Can you work these out from the model? Positions are in its coordinate system, mm. A direction names the side the tool comes from. Round coordinates to 2 decimals unless told otherwise and drop trailing zeros. Write each loop counter-clockwise with the first axis right and the second up, starting at its lowest first coordinate (ties: lowest second). Pieces come first, ordered by that corner, then holes.
Q1. Please list where these lines run through material, in increasing order: line 1 along Y through (x, z) = (-4.25, -0.75); line 2 along Y through (x, z) = (-9, -0.45); line 3 along Z through (x, y) = (4, -7.5).
Q2. For faces 1 (the conical face through (12.996, -13.063, -0.285)), 2 (the flat face through (-0.508, 2.215, -0.493)), which set-ups out of +Z, -Z, +X, -X, +Y, -Y let a thin tool reach every point of the face, with its end or its side?
Q3. If we section it at B-B (x = 5): Please give me the cut outline in (y, z), plus the area to 3 significant figures.
Q4. I'm going to push flat-ended pins straight in: pin 1 Ø8 at (x, y) = (2.5, 6) entering from +Z; pin 2 Ø0.5 at (y, z) = (7, -0.5) entering from -X; pin 3 Ø0.5 at (y, z) = (-5, -0.5) entering from +X; pin 4 Ø0.8 at (y, z) = (5, -0.5) entering from +X. Where does each tip first touch, or does it pass through?
Q5. If we section it at C-C (z = -1.5): Please give me the cut outline in (x, y).
Q6. If we section it at D-D (x = -8.25): Please give me the cut outline in (y, z).
Q7. If we section it at A-A (y = 2.25): Please give me the cut outline in (x, z), plus the area to 3 significant figures.
Q8. We'd pull the mould along X, two halves only. Please class faces 3 (the flat face through (-0.24, -2.57, -0.49)), 4 (the cylindrical face through (13, 14, -3)), 5 (the cylindrical face through (-13, -14, -3)), 6 (the flat face through (0, 3, 0)): +X half, -X half, draft (parallel to the pull), parting line (faces both ways), or undercut.
from build123d import *

# Parameters (mm, degrees)
SKETCH1_W             = 30
SKETCH1_H             = 30
BOSS_EXTRUDE1_DEPTH   = 5
SKETCH1_3_OUTSIDE_W   = 40.544
SKETCH1_3_OUTSIDE_H   = 40.544
SKETCH1_3_OUTSIDE_W_2 = 30
SKETCH1_3_OUTSIDE_H_2 = 30
CUT_EXTRUDE1_DEPTH    = 1
FILLET1_R             = 5
CHAMFER1_SIZE         = 1


with BuildPart() as part:
    # Sketch1 → Boss-Extrude1 (new body)
    with BuildSketch(Plane(origin=(0, 0, 0), x_dir=(0, 1, 0), z_dir=(0, 0, 1))):
        Rectangle(SKETCH1_W, SKETCH1_H)
    extrude(amount=-BOSS_EXTRUDE1_DEPTH)

    # Sketch1<3> outside → Cut-Extrude1 (cut)
    # profile 1 of 2: a face of its own
    with BuildSketch(Plane(origin=(0, 0, 0), x_dir=(0, 1, 0), z_dir=(0, 0, 1))):
        Rectangle(SKETCH1_3_OUTSIDE_W, SKETCH1_3_OUTSIDE_H)
        Rectangle(SKETCH1_3_OUTSIDE_W_2, SKETCH1_3_OUTSIDE_H_2, mode=Mode.SUBTRACT)
    # profile 2 of 2: a face of its own
    with BuildSketch(Plane(origin=(0, 0, 0), x_dir=(0, 1, 0), z_dir=(0, 0, 1))):
        Polygon((7.730978261, -10), (5.072463768, -10), (4.769021739, 2.68115942), (4.637681159, 7.232789855), (3.691123188, 4.524456522), (0.697463768, -3.623188406), (-1.186594203, -3.623188406), (-3.994565217, 4.216485507), (-4.927536232, 7.232789855), (-4.990942029, 2.463768116), (-5.362318841, -10), (-7.930253623, -10), (-6.933876812, 10), (-3.704710145, 10), (-1.014492754, 2.255434783), (-0.144927536, -0.357789855), (0.711050725, 2.255434783), (3.582427536, 10), (6.897644928, 10), align=None)
    extrude(amount=-CUT_EXTRUDE1_DEPTH, mode=Mode.SUBTRACT)

    # Fillet1
    fillet1_edges = [part.edges().sort_by_distance(p)[0] for p in [
        (15, 15, -2.5),
        (-15, 15, -2.5),
        (-15, -15, -2.5),
        (15, -15, -2.5),
    ]]
    fillet(fillet1_edges, radius=FILLET1_R)

    # Chamfer1
    chamfer1_edges = [part.edges().sort_by_distance(p)[0] for p in [
        (0, 15, 0),
        (15, 0, 0),
        (-15, 0, 0),
        (0, -15, 0),
        (-13.535533906, -13.535533906, 0),
        (13.535533906, -13.535533906, 0),
        (13.535533906, 13.535533906, 0),
        (-13.535533906, 13.535533906, 0),
    ]]
    chamfer(chamfer1_edges, length=CHAMFER1_SIZE)


solid = part.part
A:
1. line 1: y = -14.75 to -7.22, -4.97 to -4, -1.71 to 1.45, 3.59 to 4.72, 7.14 to 14.75
1. line 2: y = -14.45 to -6.98, -3.36 to 3.21, 6.94 to 14.45
1. line 3: z = -5 to -1
2. face 1: +Z, +X, -Y
2. face 2: +Z
3. outline: (-15, -5) - (15, -5) - (15, -1) - (14, 0) - (7.52, 0) - (7.52, -1) - (4.95, -1) - (4.95, 0) - (-5.21, 0) - (-5.21, -1) - (-7.68, -1) - (-7.68, 0) - (-14, 0) - (-15, -1) - close
3. area: 144 mm2
4. pin 1: stops at z = 0
4. pin 2: stops at x = -14.75
4. pin 3: stops at x = 14.75
4. pin 4: stops at x = 14.9
5. outline: (-15, -10) arc R5 ccw to (-10, -15) - (10, -15) arc R5 ccw to (15, -10) - (15, 10) arc R5 ccw to (10, 15) - (-10, 15) arc R5 ccw to (-15, 10) - close
6. outline: (-15, -5) - (15, -5) - (15, -1) - (14, 0) - (6.97, 0) - (6.97, -1) - (2.93, -1) - (2.93, 0) - (-3.1, 0) - (-3.1, -1) - (-7.02, -1) - (-7.02, 0) - (-14, 0) - (-15, -1) - close
7. outline: (-15, -5) - (15, -5) - (15, -1) - (14, 0) - (-0.6, 0) - (-0.6, -1) - (-6.41, -1) - (-6.41, 0) - (-14, 0) - (-15, -1) - close
7. area: 143 mm2
8. face 3: undercut
8. face 4: +X half
8. face 5: -X half
8. face 6: draft
